Work out the finished part from the listing and answer in its coordinate system (mm). A direction names the side the tool comes from. Coordinates: 2 decimals unless noted, no trailing zeros. Loops run counter-clockwise (first coordinate to the right, second up) from the corner with the lowest first, then second, coordinate; pieces in that order, holes last. Notation, with made-up numbers: (32, -23.5) -> (52, -23.5) arc R26 cw to (52, -3.5) -> close; hole circle Ø9 at (53, -17.5). An arc over 180 degrees is marked (long way). One line per question, with ' | ' between items.
```python
from build123d import *

# Parameters (mm, degrees)
EXTRUDE_1_DEPTH     = 50
SKETCH_3_R          = 6.5
SKETCH_3_R_2        = 1.5
CUT_EXTRUDE_1_DEPTH = 50
SKETCH_4_R          = 2.5
CUT_EXTRUDE_2_DEPTH = 50


with BuildPart() as part:
    # 草图2 → 凸台-拉伸1 (new body)
    with BuildSketch(Plane(origin=(0, 0, 0), x_dir=(0, 0, -1), z_dir=(1, 0, 0))):
        Polygon((0, 0), (50, 0), (50, 50), (48, 50), (48, 2), (0, 2), align=None)
    extrude(amount=EXTRUDE_1_DEPTH)

    # 草图3 → 切除-拉伸1 (cut)
    with BuildSketch(Plane(origin=(0, 0, -50), x_dir=(-1, 0, 0), z_dir=(0, 0, -1))):
        with Locations((-25, 26)):
            Circle(SKETCH_3_R)
        with Locations((-25, 35.5)):
            Circle(SKETCH_3_R_2)
        with Locations((-16.772758664, 30.75)):
            Circle(SKETCH_3_R_2)
        with Locations((-16.772758664, 21.25)):
            Circle(SKETCH_3_R_2)
        with Locations((-25, 16.5)):
            Circle(SKETCH_3_R_2)
        with Locations((-33.227241336, 21.25)):
            Circle(SKETCH_3_R_2)
        with Locations((-33.227241336, 30.75)):
            Circle(SKETCH_3_R_2)
    extrude(amount=-CUT_EXTRUDE_1_DEPTH, mode=Mode.SUBTRACT)

    # 草图4 → 切除-拉伸2 (cut)
    with BuildSketch(Plane.XZ):
        with Locations(Location((10, -10, 0), (0, 0, 270))):
            Circle(SKETCH_4_R)
        with Locations(Location((40, -10, 0), (0, 0, 270))):
            Circle(SKETCH_4_R)
        with Locations(Location((10, -40, 0), (0, 0, 270))):
            Circle(SKETCH_4_R)
        with Locations(Location((40, -40, 0), (0, 0, 270))):
            Circle(SKETCH_4_R)
    extrude(amount=-CUT_EXTRUDE_2_DEPTH, mode=Mode.SUBTRACT)


solid = part.part
```
1) For faces 1 (the face through (16.968, 32.237, -49.014)), 2 (the face through (25, 2, -24)), determine the directions among +Z, -Z, +X, -X, +Y, -Y from which every point of the face is accessible in a straight line to the end or side of a thin tool.
Check values:
face 1: +Z, -Z | face 2: +Z, +X, -X, +Y
2) Find the intervals of material crossed by line 1 along Y through (x, z) = (25, -49); line 2 along Z through (x, y) = (19, 33); line 3 along Y through (x, z) = (28, -25.5), in increasing order.
Check values:
line 1: y = 0 to 15, 18 to 19.5, 32.5 to 34, 37 to 50 | line 2: z = -50 to -48 | line 3: y = 0 to 2
3) Find section C-C (y = 35.5). Write down the section's boundary in (x, z).
Check values:
outline: (0, -50) -> (23.5, -50) -> (23.5, -48) -> (0, -48) -> close; (26.5, -50) -> (50, -50) -> (50, -48) -> (26.5, -48) -> close
4) Find section A-A (x = 40). Write down the section's boundary in (y, z).
Check values:
outline: (0, -50) -> (50, -50) -> (50, -48) -> (2, -48) -> (2, -42.5) -> (0, -42.5) -> close; (0, -37.5) -> (2, -37.5) -> (2, -12.5) -> (0, -12.5) -> close; (0, -7.5) -> (2, -7.5) -> (2, 0) -> (0, 0) -> close
5) Flat-ended cylindrical pins translate along their axes: pin 1 (1 mm diameter, centred on x = 5, z = -14.5, fed in from +Y); pin 2 (4 mm diameter, centred on x = 25, y = 16.5, fed in from +Z). Find the tip coordinate at first contact, or state that the pin passes through.
Check values:
pin 1: stops at y = 2 | pin 2: stops at z = -48
6) The mould has two halves that part along Z. Classify faces 3 (the face through (19, 32, -48)), 4 (the face through (37.56, 0.99, -9.46)), 5 (the face through (0, 1, -36)): released by +Z, released by -Z, zero draft, split by the parting line, or undercut.
Check values:
face 3: released by +Z | face 4: undercut | face 5: zero draft
7) Find section D-D (x = 25). Write down the section's boundary in (y, z).
Check values:
outline: (0, -50) -> (15, -50) -> (15, -48) -> (2, -48) -> (2, 0) -> (0, 0) -> close; (18, -50) -> (19.5, -50) -> (19.5, -48) -> (18, -48) -> close; (32.5, -50) -> (34, -50) -> (34, -48) -> (32.5, -48) -> close; (37, -50) -> (50, -50) -> (50, -48) -> (37, -48) -> close
8) Find section B-B (z = -10). Write down the section's boundary in (x, y).
Check values:
outline: (0, 0) -> (7.5, 0) -> (7.5, 2) -> (0, 2) -> close; (12.5, 0) -> (37.5, 0) -> (37.5, 2) -> (12.5, 2) -> close; (42.5, 0) -> (50, 0) -> (50, 2) -> (42.5, 2) -> close
